Build history of the part. All positions in model axes, mm. Give positions to 0.01 mm unless a question says otherwise; leave off trailing zeros. Order: outer loops, then holes, each group sorted by start corner. A loop starts at its lowest first (then second) coordinate and runs counter-clockwise, first axis right, second up. Notation, with made-up numbers: (52, 41.5) - (82, 41.5) arc R19 cw to (82, 49.5) - close; hole circle Ø1 at (3.5, 56). An arc over 180 degrees is marked (long way). Write each question's results on one line, items separated by ' | '. Start each with the question number.
1) Two-plate mould, pull along Y, no slides. Class faces 1 (the face through (28, -65, 0)), 2 (the face through (-13.85, -67.22, 2.54)), 3 (the face through (-399.988, -364.992, 2.465)), 4 (the face through (-2.3, 369.4, 2.5)): +Y half, -Y half, draft (parallel to the pull), parting line (faces both ways), or undercut.
2) Drop flat-ended pins along their axis: pin 1 Ø1 at (y, z) = (-106, 4.5) entering from -X; pin 2 Ø24 at (x, y) = (174.87, 224.02) entering from -Z; pin 3 Ø2 at (x, z) = (-98.5, 0.5) entering from -Y; pin 4 Ø3 at (x, z) = (-229.5, 3.5) entering from +Y. Give the stop position or say it passes through.
3) Drill centre lines: line 1 along Y through (x, z) = (350, 3); line 2 along X through (y, z) = (-183, 1.1); line 3 along Y through (x, z) = (-251, 3.3). Where is each one in solid material? Low to high. Write a range as from..to.
4) Cut at A-A on x = 140. List the corners of the cut face in (y, z), plus the area to 3 significant figures.
5) Cut at B-B on z = 2.8. State how many separate pieces and enclosed holes the cut face has, plus the area to 3 significant figures.
from build123d import *

# Parameters (mm, degrees)
BOSS_EXTRUDE2_DEPTH = 5
SKETCH2_R           = 19.127666072
SKETCH2_R_2         = 17.449363928
SKETCH2_R_3         = 20.149507696
CUT_EXTRUDE1_DEPTH  = 60


with BuildPart() as part:
    # Sketch1 → Boss-Extrude2 (new body)
    with BuildSketch(Plane.XY):
        with BuildLine():
            Line((-75, 383.908045977), (-89.272030651, -15.708812261))
            Line((-89.272030651, -15.708812261), (-282.566478984, -209.003260593))
            ThreePointArc((-282.566478984, -209.003260593), (-277.81350135, -276.433117622), (-210.383644321, -271.680139987))
            Line((-210.383644321, -271.680139987), (-93.90556369, -145.447737332))
            Line((-93.90556369, -145.447737332), (-100, -316.091954023))
            Line((-100, -316.091954023), (-350, -316.091954023))
            ThreePointArc((-350, -316.091954023), (-400, -366.091954023), (-350, -416.091954023))
            Line((-350, -416.091954023), (-100, -416.091954023))
            ThreePointArc((-100, -416.091954023), (0, -457.51331026), (100, -416.091954023))
            Line((100, -416.091954023), (350, -416.091954023))
            ThreePointArc((350, -416.091954023), (400, -366.091954023), (350, -316.091954023))
            Line((350, -316.091954023), (100, -316.091954023))
            Line((100, -316.091954023), (86.907181572, 50.506961966))
            Line((86.907181572, 50.506961966), (350, 335.632183908))
            ThreePointArc((350, 335.632183908), (333.983863171, 399.924182806), (269.691864273, 383.908045977))
            Line((269.691864273, 383.908045977), (82.685549205, 168.712668231))
            Line((82.685549205, 168.712668231), (75, 383.908045977))
            ThreePointArc((75, 383.908045977), (0, 458.908045977), (-75, 383.908045977))
        make_face()
    extrude(amount=BOSS_EXTRUDE2_DEPTH)

    # Sketch2 → Cut-Extrude1 (cut)
    with BuildSketch(Plane.XY.offset(5)):
        with Locations((-280, -366.091954023)):
            Circle(SKETCH2_R)
        with Locations((-210, -366.091954023)):
            Circle(SKETCH2_R)
        with Locations((-350, -366.091954023)):
            Circle(SKETCH2_R)
        with Locations((-140, -366.091954023)):
            Circle(SKETCH2_R)
        with Locations((-70, -366.091954023)):
            Circle(SKETCH2_R)
        with Locations((0, -366.091954023)):
            Circle(SKETCH2_R)
        with Locations((70, -366.091954023)):
            Circle(SKETCH2_R)
        with Locations((140, -366.091954023)):
            Circle(SKETCH2_R)
        with Locations((210, -366.091954023)):
            Circle(SKETCH2_R)
        with Locations((280, -366.091954023)):
            Circle(SKETCH2_R)
        with Locations((350, -366.091954023)):
            Circle(SKETCH2_R)
        with Locations((0, 415.848503824)):
            Circle(SKETCH2_R_2)
        with Locations((0, 352.103321769)):
            Circle(SKETCH2_R_2)
        with Locations((0, 290.357789176)):
            Circle(SKETCH2_R_2)
        with Locations((0, 223.223112333)):
            Circle(SKETCH2_R_2)
        with Locations((0, 150.590486971)):
            Circle(SKETCH2_R_2)
        with Locations((0, -56.606498774)):
            Circle(SKETCH2_R_2)
        with Locations((0, -117.853104706)):
            Circle(SKETCH2_R_2)
        with Locations((0, -181.842565513)):
            Circle(SKETCH2_R_2)
        with Locations((0, -253.635619101)):
            Circle(SKETCH2_R_2)
        with Locations((0, -311.755022078)):
            Circle(SKETCH2_R_2)
        with Locations((0, -427.95103023)):
            Circle(SKETCH2_R_2)
        with Locations((-245.128862806, -240.299431579)):
            Circle(SKETCH2_R_3)
        with Locations((-204.579359837, -195.470941049)):
            Circle(SKETCH2_R_3)
        with Locations((-151.934117667, -137.270308063)):
            Circle(SKETCH2_R_3)
        with Locations((-105.128862806, -85.525927228)):
            Circle(SKETCH2_R_3)
        with Locations((-57.302051438, -32.652190104)):
            Circle(SKETCH2_R_3)
        with Locations((-10.671022438, 18.899579681)):
            Circle(SKETCH2_R_3)
        with Locations((34.871137194, 69.247577124)):
            Circle(SKETCH2_R_3)
        with Locations((80.497867488, 119.68906955)):
            Circle(SKETCH2_R_3)
        with Locations((129.746983315, 174.135199855)):
            Circle(SKETCH2_R_3)
        with Locations((174.871137194, 224.021081476)):
            Circle(SKETCH2_R_3)
        with Locations((215.441503687, 268.872637154)):
            Circle(SKETCH2_R_3)
        with Locations((258.052096157, 314.419110743)):
            Circle(SKETCH2_R_3)
        with Locations((298.226980998, 359.414981764)):
            Circle(SKETCH2_R_3)
    extrude(amount=-CUT_EXTRUDE1_DEPTH, mode=Mode.SUBTRACT)


solid = part.part
Results:
1) face 1: draft | face 2: undercut | face 3: parting line | face 4: undercut
2) pin 1: x = -180.06 | pin 2: through | pin 3: y = -418.53 | pin 4: y = -154.44
3) line 1: -416.09..-385.22, -346.96..-316.09, 335.63..383.91 | line 2: -256.56..-220.41, -188.75..-128.56, -95.25..-17.41, 17.41..95.25 | line 3: -416.09..-316.09, -287.93..-259.57, -221.02..-177.44
4) outline: (-416.09, 0) - (-385.22, 0) - (-385.22, 5) - (-416.09, 5) - close; (-346.96, 0) - (-316.09, 0) - (-316.09, 5) - (-346.96, 5) - close; (108.05, 0) - (156.79, 0) - (156.79, 5) - (108.05, 5) - close; (191.48, 0) - (234.67, 0) - (234.67, 5) - (191.48, 5) - close | area: 768 mm^2
5) separate pieces: 1 | enclosed holes: 35 | area: 232,000 mm^2
